Design review of the part shown in the three views and the two pictorial views. Dimensions are in mm from the part's minimum x, y and z. Round coordinates to 2 decimals unless told otherwise and drop trailing zeros. Loops run counter-clockwise (first coordinate to the right, second up) from the corner with the lowest first, then second, coordinate; pieces in that order, holes last.
1. Consider section C-C on y = 19.75. State the section outline as (x, z) points.
2. Consider section A-A on z = 4.25. State the section outline as (x, y) points.
3. Draft analysis for pull direction Y (two halves, no side actions). For the marked faces 1, 2 and 3, state which applies: released by +Y, released by -Y, zero draft, split by the parting line, or undercut.
4. To check wall thickness, follow line 1 along Y through (x, z) = (12, 3.45); line 2 along X through (y, z) = (6.5, 3.4); line 3 along Z through (x, y) = (43, 25). State the ranges of each line that lie inside material, in increasing order.
5. Consider section B-B on x = 34.5. State the section outline as (y, z) points, then the cut area to 3 significant figures.
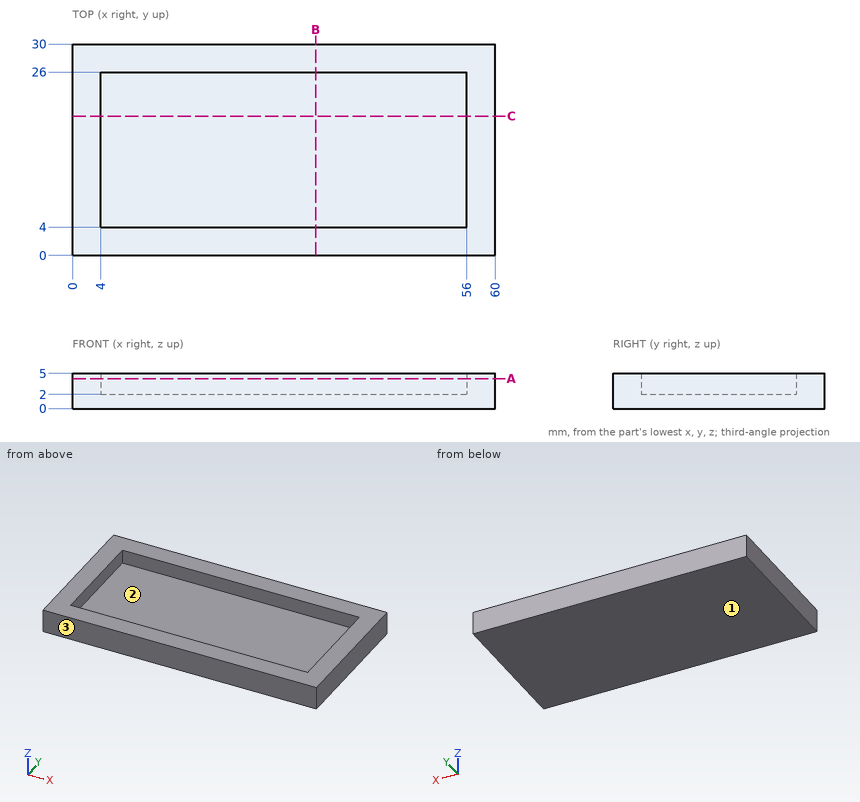
Resolved:
1. outline: (0, 0) - (60, 0) - (60, 5) - (56, 5) - (56, 2) - (4, 2) - (4, 5) - (0, 5) - close
2. outline: (0, 0) - (60, 0) - (60, 30) - (0, 30) - close; hole (4, 4) - (56, 4) - (56, 26) - (4, 26) - close
3. face 1: zero draft
3. face 2: undercut
3. face 3: released by -Y
4. line 1: y = 0 to 4, 26 to 30
4. line 2: x = 0 to 4, 56 to 60
4. line 3: z = 0 to 2
5. outline: (0, 0) - (30, 0) - (30, 5) - (26, 5) - (26, 2) - (4, 2) - (4, 5) - (0, 5) - close
5. area: 84.0 mm2
